```python
from build123d import *

# Parameters (mm, degrees)
EXTRUSION1_DEPTH = 28.5
ESQUISSE2_R      = 1.5
EXTRUSION2_DEPTH = 47.5
ESQUISSE3_R      = 1.5
EXTRUSION3_DEPTH = 10


with BuildPart() as part:
    # Esquisse1 → Extrusion1 (new body)
    with BuildSketch(Plane.XY):
        Polygon((-16.977160064, 3.864315789), (-16.977160064, -16.135684211), (3.022839936, -16.135684211), (3.022839936, -14.635684211), (-15.477160064, -14.635684211), (-15.477160064, 3.864315789), align=None)
    extrude(amount=EXTRUSION1_DEPTH)

    # Esquisse2 → Extrusion2 (cut)
    with BuildSketch(Plane.ZY.offset(16.977160064)):
        with Locations(Location((21, -6.135684211, 0), (0, 0, 270))):
            Circle(ESQUISSE2_R)
        with Locations(Location((7.5, -6.135684211, 0), (0, 0, 270))):
            Circle(ESQUISSE2_R)
    extrude(amount=-EXTRUSION2_DEPTH, mode=Mode.SUBTRACT)

    # Esquisse3 → Extrusion3 (cut)
    with BuildSketch(Plane.XZ.offset(16.135684211)):
        with Locations(Location((-6.977160064, 7.5, 0), (0, 0, 270))):
            Circle(ESQUISSE3_R)
        with Locations(Location((-6.977160064, 21, 0), (0, 0, 270))):
            Circle(ESQUISSE3_R)
    extrude(amount=-EXTRUSION3_DEPTH, mode=Mode.SUBTRACT)


solid = part.part
```
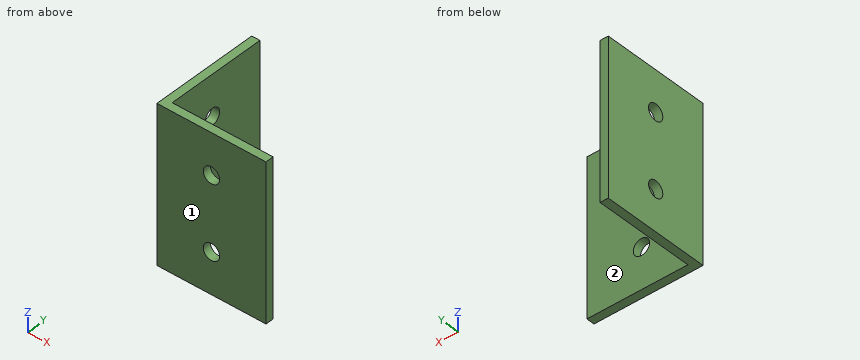
Geometry check sheet. Reference: the model listing, model coordinates, mm. Face numbers are marked on the shaded views. A direction names the side the tool comes from. Coordinates: 2 decimals unless noted, no trailing zeros. Order: outer loops, then holes, each group sorted by start corner. A loop starts at its lowest first (then second) coordinate and runs counter-clockwise, first axis right, second up. Notation, with made-up numbers: M -11,-5 L 18,-5 A10 ccw 18,13 Z; hole C 79,6 d10. An arc over 180 degrees is marked long. Answer as a JSON object with one key per item and string values.
Q1. Cross-section at B-B on x = -7.75. Record the cut outline in (y, z), and give its area (3 significant figures).
Results are:
{"outline": "M -16.14,0 L -14.64,0 L -14.64,6.21 L -16.14,6.21 Z; M -16.14,8.79 L -14.64,8.79 L -14.64,19.71 L -16.14,19.71 Z; M -16.14,22.29 L -14.64,22.29 L -14.64,28.5 L -16.14,28.5 Z", "area": "35.0 mm²"}
Q2. Cross-section at A-A on z = 21. Record the cut outline in (x, y).
Results are:
{"outline": "M -16.98,-16.14 L -8.48,-16.14 L -8.48,-14.64 L -15.48,-14.64 L -15.48,-7.64 L -16.98,-7.64 Z; M -16.98,-4.64 L -15.48,-4.64 L -15.48,3.86 L -16.98,3.86 Z; M -5.48,-16.14 L 3.02,-16.14 L 3.02,-14.64 L -5.48,-14.64 Z"}
Q3. Tool access check on the marked faces 1 and 2. Record the directions out of +Z, -Z, +X, -X, +Y, -Y that give a thin tool (end or side, any length) a straight path to the whole face; none if there is none.
Results are:
{"face 1": "+Z, -Z, +X, -X, -Y", "face 2": "+Z, -Z, +X, +Y"}
Q4. Scan lines: line 1 (X direction, y = -15.25, z = 7.5); line 2 (X direction, y = 0, z = 5.75); line 3 (Y direction, x = -3.75, z = 19.75). Record each from-to range of solid material in increasing order.
Results are:
{"line 1": "x = -16.98 to -8.48, -5.48 to 3.02", "line 2": "x = -16.98 to -15.48", "line 3": "y = -16.14 to -14.64"}
Q5. Depth check by flat-ended pin: pin 1 Ø10 at (x, y) = (-7, -9.5) entering from +Z; pin 2 Ø3 at (y, z) = (-2.5, 23) entering from +X; pin 3 Ø3.5 at (x, z) = (-6.98, 7.5) entering from +Y. Enter the tip coordinate at first touch or a pass-through.
Results are:
{"pin 1": "passes through", "pin 2": "stops at x = -15.48", "pin 3": "stops at y = -14.64"}
Q6. Cross-section at C-C on y = -11. Record the cut outline in (x, z), and give its area (4 significant figures).
Results are:
{"outline": "M -16.98,0 L -15.48,0 L -15.48,28.5 L -16.98,28.5 Z", "area": "42.75 mm²"}
Q7. Cross-section at D-D on z = 6.5. Record the cut outline in (x, y), and give its area (3 significant figures).
Results are:
{"outline": "M -16.98,-16.14 L -8.1,-16.14 L -8.1,-14.64 L -15.48,-14.64 L -15.48,-7.25 L -16.98,-7.25 Z; M -16.98,-5.02 L -15.48,-5.02 L -15.48,3.86 L -16.98,3.86 Z; M -5.86,-16.14 L 3.02,-16.14 L 3.02,-14.64 L -5.86,-14.64 Z", "area": "51.0 mm²"}
